Geometry: final body of the model. Coordinates: model frame, mm. A direction names the side the tool comes from. Coordinates: 2 decimals unless noted, no trailing zeros. Loops run counter-clockwise (first coordinate to the right, second up) from the corner with the lowest first, then second, coordinate; pieces in that order, holes last. Notation, with made-up numbers: (86.5, 45.25) - (114.5, 45.25) arc R14 cw to (114.5, 67.25) - close; hole circle Ø6 at (14.5, 25.25). An arc over 180 degrees is marked (long way). Put each result on its own line as item: value. Start each with the question number.
1) Reachability of faces 4 (the flat face through (21, 0, 8)), 5 (the flat face through (0, 0, -17)), 6 (the cylindrical face through (21.465, -4.214, -2.192)) from +Z, -Z, +X, -X, +Y, -Y: full face, straight path, thin tool, end or side. Return the list, or none.
2) Section A-A on y = 0. Output: boundary loops of the cut face in (x, z), and give its area (3 significant figures).
3) Section C-C on x = 11.5. Output: boundary loops of the cut face in (y, z).
4) Contact query for flat-ended pins moving along their axis: pin 1 Ø1.5 at (x, z) = (8.5, -7) entering from +Y; pin 2 Ø3 at (x, z) = (17.5, 8.5) entering from -Y; pin 3 Ø8 at (y, z) = (-2.5, -12) entering from +X. Output: stop coordinate, or through.
5) Draft query along Z for faces 1 (the flat face through (24, -1, -3)), 2 (the cylindrical face through (23.46, -6.59, 1.46)), 3 (the flat face through (26, -1, -3)). Return one class per face: +Z half, -Z half, draft (parallel to the pull), parting line (faces both ways), or undercut.
6) Material intervals for line 1 along Y through (x, z) = (20.25, 0); line 2 along Y through (x, z) = (12, 0); line 3 along X through (y, z) = (3.5, 7.5), sorted ascending. Write a range as from..to.
7) Section D-D on z = -15. Output: boundary loops of the cut face in (x, y), and give its area (3 significant figures).
```python
from build123d import *

# Parameters (mm, degrees)
SKETCH1_R           = 18.5
BOSS_EXTRUDE1_DEPTH = 21
SKETCH2_R           = 6.75
BOSS_EXTRUDE2_DEPTH = 5
SHELL1_T            = -2
SKETCH3_R           = 3
CUT_EXTRUDE1_DEPTH  = 5


with BuildPart() as part:
    # Sketch1 → Boss-Extrude1 (new body)
    with BuildSketch(Plane(origin=(0, 0, 0), x_dir=(0, 0, -1), z_dir=(1, 0, 0))):
        with Locations(Location((0, 0, 0), (0, 0, 180))):
            Circle(SKETCH1_R)
    extrude(amount=BOSS_EXTRUDE1_DEPTH)

    # Sketch2 → Boss-Extrude2 (add)
    with BuildSketch(Plane(origin=(21, 0, 0), x_dir=(0, 0, -1), z_dir=(1, 0, 0))):
        Circle(SKETCH2_R)
    extrude(amount=BOSS_EXTRUDE2_DEPTH)

    # Shell1
    shell1_openings = [part.faces().sort_by_distance(p)[0] for p in [
        (0, 0, 0),
    ]]
    offset(amount=SHELL1_T, openings=shell1_openings, kind=Kind.INTERSECTION)

    # Sketch3 → Cut-Extrude1 (cut)
    with BuildSketch(Plane(origin=(26, 0, 0), x_dir=(0, 0, -1), z_dir=(1, 0, 0))):
        Circle(SKETCH3_R)
    extrude(amount=-CUT_EXTRUDE1_DEPTH, mode=Mode.SUBTRACT)


solid = part.part
```
Answer block:
1. face 4: +X
1. face 5: +Z, -Z, -X, +Y, -Y
1. face 6: -X
2. outline: (0, -18.5) - (21, -18.5) - (21, -6.75) - (26, -6.75) - (26, -3) - (24, -3) - (24, -4.75) - (19, -4.75) - (19, -16.5) - (0, -16.5) - close; (0, 16.5) - (19, 16.5) - (19, 4.75) - (24, 4.75) - (24, 3) - (26, 3) - (26, 6.75) - (21, 6.75) - (21, 18.5) - (0, 18.5) - close
2. area: 158 mm²
3. outline: circle Ø37 at (0, 0); hole circle Ø33 at (0, 0)
4. pin 1: stops at y = 17.41
4. pin 2: stops at y = -17.12
4. pin 3: stops at x = 21
5. face 1: undercut
5. face 2: parting line
5. face 3: draft
6. line 1: y = -18.5..-4.75, 4.75..18.5
6. line 2: y = -18.5..-16.5, 16.5..18.5
6. line 3: x = 19..21
7. outline: (0, -10.83) - (21, -10.83) - (21, 10.83) - (0, 10.83) - (0, 6.87) - (19, 6.87) - (19, -6.87) - (0, -6.87) - close
7. area: 194 mm²
